from build123d import *

# Parameters (mm, degrees)
F1_DEPTH = 5


with BuildPart() as f1:
    # F0 (on Top) → F1 (new body)
    with BuildSketch(Plane.XY):
        Polygon((-106, 0), (0, 0), (0, 25), (-165, 25), (-165, 0), (-143, 0), (-143, -6), (-136, -6), (-136, 0), (-113, 0), (-113, -6), (-106, -6), align=None)
    extrude(amount=F1_DEPTH)

    # F2: F1 across face


with BuildPart() as f1_1:
    add(f1.part)
    add(f1.part.mirror(Plane(origin=(0, 12.5, 2.5), x_dir=(0, 1, 0), z_dir=(1, 0, 0))))


solid = f1_1.part
Can you work these out from the model? Positions are in its coordinate system, mm. A direction names the side the tool comes from. Coordinates: 2 decimals unless noted, no trailing zeros. Order: outer loops, then holes, each group sorted by start corner. A loop starts at its lowest first (then second) coordinate and runs counter-clockwise, first axis right, second up. Notation, with made-up numbers: M 20.5,57 L 39.5,57 A23 ccw 39.5,94 Z; hole C -28,68.25 d2. An arc over 180 degrees is marked long. Write item = value, one per line.
(1) If we mould it in two halves opening along X, with no side actions, what happens to faces 1 (the face through (106, -3, 2)), 2 (the face through (-165, 13, 2)), 3 (the face through (-110, -6, 2))? For each: pulls with the +X half, pulls with the -X half, needs draft (parallel to the pull), parting line crosses it, or undercut.
Results are:
face_1 = undercut
face_2 = pulls with the -X half
face_3 = needs draft
(2) I need wall thicknesses on line 1 along X through (y, z) = (-3, 0.4); line 2 along Y through (x, z) = (-70.5, 3). Which ranges of each line are inside material? Lowest first, please. Write a range as [from, to].
Results are:
line_1 = [-143, -136], [-113, -106], [106, 113], [136, 143]
line_2 = [0, 25]
(3) Suppose I cut it at B-B on x = -46.5. Please give me the cut outline in (y, z), plus the area to 3 significant figures.
Results are:
outline = M 0,0 L 25,0 L 25,5 L 0,5 Z
area = 125 mm2
(4) For faces 4 (the face through (143, -3, 2)), 5 (the face through (-154, 0, 2)), 6 (the face through (136, -3, 2)), which set-ups out of +Z, -Z, +X, -X, +Y, -Y let a thin tool reach every point of the face, with its end or its side?
Results are:
face_4 = +Z, -Z, +X, -Y
face_5 = +Z, -Z, -X, -Y
face_6 = +Z, -Z, -Y
(5) Suppose I cut it at A-A on z = 3.8. Please give me the cut outline in (x, y).
Results are:
outline = M -165,0 L -143,0 L -143,-6 L -136,-6 L -136,0 L -113,0 L -113,-6 L -106,-6 L -106,0 L 106,0 L 106,-6 L 113,-6 L 113,0 L 136,0 L 136,-6 L 143,-6 L 143,0 L 165,0 L 165,25 L -165,25 Z
(6) For pin 1 Ø2.5 at (y, z) = (-1.5, 2.5) entering from +X; pin 2 Ø3 at (x, z) = (38.5, 1.5) entering from -Y; pin 3 Ø1.5 at (y, z) = (-4.5, 1.5) entering from -X, each with a flat end and sliding along its axis, tell me the tip position at first contact or that it passes through.
Results are:
pin_1 = 143
pin_2 = 0
pin_3 = -143
